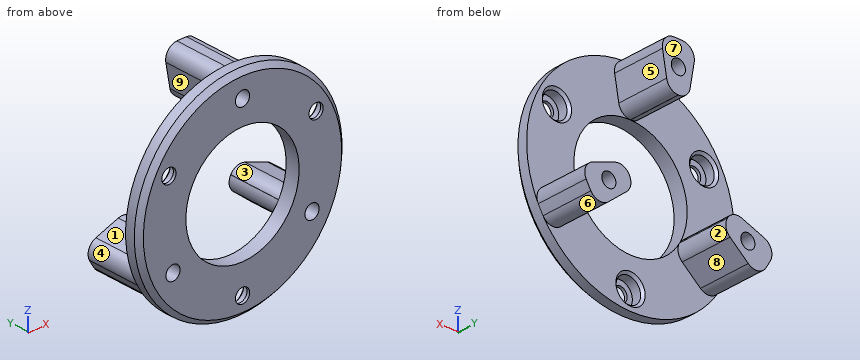
from build123d import *
from build123d.topology import SkipClean

# Parameters (mm, degrees)
SKETCH1_R           = 22
SKETCH1_R_2         = 12
BOSS_EXTRUDE1_DEPTH = 3
SKETCH3_R           = 1.5
CUT_EXTRUDE2_DEPTH  = 32.256999216
SKETCH5_R           = 2.6
CUT_EXTRUDE3_DEPTH  = 2.4
CIRPATTERN1_COUNT   = 3
SKETCH4_R           = 1.5
BOSS_EXTRUDE2_DEPTH = 11
CIRPATTERN2_COUNT   = 3
FILLET1_R           = 2.5
CHAMFER1_SIZE       = 0.5
CHAMFER2_SIZE       = 1


with BuildPart() as part:
    # Sketch1 → Boss-Extrude1 (new body)
    with BuildSketch(Plane(origin=(0, 0, 0), x_dir=(1, 0, 0), z_dir=(0, 1, 0))):
        with Locations(Location((0, 0, 0), (0, 0, 270))):
            Circle(SKETCH1_R)
        with Locations(Location((0, 0, 0), (0, 0, 270))):
            Circle(SKETCH1_R_2, mode=Mode.SUBTRACT)
    extrude(amount=BOSS_EXTRUDE1_DEPTH)

    # Sketch3 → Cut-Extrude2 (cut, through all)
    with BuildSketch(Plane(origin=(0, 3, 0), x_dir=(1, 0, 0), z_dir=(0, 1, 0))):
        with Locations(Location((14.722431864, 8.5, 0), (0, 0, 270))):
            Circle(SKETCH3_R)
        with Locations(Location((0, 18, 0), (0, 0, 270))):
            Circle(SKETCH3_R)
    cut_extrude2 = extrude(amount=-CUT_EXTRUDE2_DEPTH, mode=Mode.SUBTRACT)

    # Sketch5 → Cut-Extrude3 (cut)
    with BuildSketch(Plane(origin=(0, 3, 0), x_dir=(1, 0, 0), z_dir=(0, 1, 0))):
        with Locations(Location((0, 18, 0), (0, 0, 270))):
            Circle(SKETCH5_R)
    cut_extrude3 = extrude(amount=-CUT_EXTRUDE3_DEPTH, mode=Mode.SUBTRACT)

    # CirPattern1: Cut-Extrude2, Cut-Extrude3 ×3 about axis
    cirpattern1_axis = Axis((0, 0, 0), (0, 1, 0))
    add([cut_extrude2.rotate(cirpattern1_axis, i * 360 / CIRPATTERN1_COUNT) for i in range(1, CIRPATTERN1_COUNT)], mode=Mode.SUBTRACT)
    add([cut_extrude3.rotate(cirpattern1_axis, i * 360 / CIRPATTERN1_COUNT) for i in range(1, CIRPATTERN1_COUNT)], mode=Mode.SUBTRACT)

    # Sketch4 → Boss-Extrude2 (add)
    with SkipClean():  # the faces are left unmerged after this step: merging them gives an invalid solid
        with BuildSketch(Plane(origin=(0, 3, 0), x_dir=(1, 0, 0), z_dir=(0, 1, 0))):
            with BuildLine():
                Line((9.192533317, 7.713451316), (16.852977749, 14.141327413))
                ThreePointArc((16.852977749, 14.141327413), (19.052558883, 11), (20.673237657, 7.524443153))
                Line((20.673237657, 7.524443153), (11.276311449, 4.10424172))
                ThreePointArc((11.276311449, 4.10424172), (10.392304845, 6), (9.192533317, 7.713451316))
            make_face()
            with Locations(Location((14.722431864, 8.5, 0), (0, 0, 270))):
                Circle(SKETCH4_R, mode=Mode.SUBTRACT)
        boss_extrude2 = extrude(amount=BOSS_EXTRUDE2_DEPTH)

    # CirPattern2: Boss-Extrude2 ×3 about axis
    with SkipClean():  # the faces are left unmerged after this step: merging them gives an invalid solid
        cirpattern2_axis = Axis((0, 0, 0), (0, 1, 0))
        for i in range(1, CIRPATTERN2_COUNT):
            add(boss_extrude2.rotate(cirpattern2_axis, i * 360 / CIRPATTERN2_COUNT))

    # Fillet1
    # the kernel refuses this fillet: 2.5 mm, written as the material it takes off along each edge
    with BuildSketch(Plane(origin=(9.192533317, 3, -7.713451316), x_dir=(0.7660444431189769, 0, -0.6427876096865408), z_dir=(0, 1, 0)), Plane(origin=(-11.276311449, 3, -4.10424172), x_dir=(-0.9396926207859091, 0, -0.34202014332566705), z_dir=(0, 1, 0)), Plane(origin=(2.083778132, 3, 11.817693036), x_dir=(0.1736481776669318, 0, 0.9848077530122079), z_dir=(0, 1, 0))) as fillet1_piece_1:
        with BuildLine():
            CenterArc((2.282856857, -2.5), FILLET1_R, 90, 80.071808158)
            ThreePointArc((-0.17970467, -2.068965517), (-0.045010582, -1.03837759), (0, 0))
            Line((0, 0), (2.282856857, 0))
        make_face()
    extrude(amount=16.707142143, mode=Mode.SUBTRACT)
    with BuildSketch(Plane(origin=(11.276311449, 3, -4.10424172), x_dir=(0.9396926207859079, 0, -0.34202014332567005), z_dir=(0, 1, 0)), Plane(origin=(-9.192533317, 3, -7.713451316), x_dir=(-0.7660444431189779, 0, -0.6427876096865395), z_dir=(0, 1, 0)), Plane(origin=(-2.083778132, 3, 11.817693036), x_dir=(-0.17364817766692894, 0, 0.9848077530122082), z_dir=(0, 1, 0))) as fillet1_piece_2:
        with BuildLine():
            CenterArc((2.282856857, 2.5), FILLET1_R, 189.928191842, 80.071808158)
            ThreePointArc((-0.17970467, 2.068965517), (-0.045010582, 1.03837759), (0, 0))
            Line((0, 0), (2.282856857, 0))
        make_face()
    extrude(amount=16.707142143, mode=Mode.SUBTRACT)
    with BuildSketch(Plane(origin=(20.673237657, 3, -7.524443153), x_dir=(-0.40167516398546327, 0, -0.9157822135405619), z_dir=(0, 1, 0)), Plane(origin=(-16.852977749, 3, -14.141327413), x_dir=(-0.5922530792673408, 0, 0.8057520028509721), z_dir=(0, 1, 0)), Plane(origin=(-3.820259909, 3, 21.665770566), x_dir=(0.9939282432528036, 0, 0.11003021068958989), z_dir=(0, 1, 0))) as fillet1_piece_3:
        with BuildLine():
            CenterArc((2.66576178, 2.494836964), FILLET1_R, 176.317057086, 97.365885829)
            Line((0.170924817, 2.655425023), (0, 0))
            ThreePointArc((0, 0), (1.41317492, -0.04543472), (2.826349839, 0))
        make_face()
    extrude(amount=18.065874598, mode=Mode.SUBTRACT)
    with BuildSketch(Plane(origin=(16.852977749, 3, -14.141327413), x_dir=(0.5922530792673405, 0, 0.8057520028509723), z_dir=(0, 1, 0)), Plane(origin=(-20.673237657, 3, -7.524443153), x_dir=(0.40167516398546094, 0, -0.9157822135405629), z_dir=(0, 1, 0)), Plane(origin=(3.820259909, 3, 21.665770566), x_dir=(-0.9939282432528035, 0, 0.11003021068959112), z_dir=(0, 1, 0))) as fillet1_piece_4:
        with BuildLine():
            CenterArc((2.66576178, -2.494836964), FILLET1_R, 86.317057086, 97.365885829)
            Line((0.170924817, -2.655425023), (0, 0))
            ThreePointArc((0, 0), (1.41317492, 0.04543472), (2.826349839, 0))
        make_face()
    extrude(amount=18.065874598, mode=Mode.SUBTRACT)

    # Chamfer1
    chamfer1_edges = [part.edges().sort_by_distance(p)[0] for p in [
        (0, 3, -20.6),
        (17.840123318, 3, 10.3),
        (-17.840123318, 3, 10.3),
    ]]
    chamfer(chamfer1_edges, length=CHAMFER1_SIZE)

    # Chamfer2
    chamfer2_edges = [part.edges().sort_by_distance(p)[0] for p in [
        (0, 0, -22),
    ]]
    chamfer(chamfer2_edges, length=CHAMFER2_SIZE)


solid = part.part
Input: part model. Units: mm. Frame: model coordinates. Face numbers are marked on the shaded views. A direction names the side the tool comes from. Round coordinates to 2 decimals unless told otherwise and drop trailing zeros. Answer as CSV lines item,"result". Start each with the question number.
(1) Reachability of the marked faces 1, 2, 3, 4 and 5 from +Z, -Z, +X, -X, +Y, -Y: full face, straight path, thin tool, end or side. Return the list, or none.
(2) Line query: line 1 (X direction, y = 1, z = -8); line 2 (X direction, y = 1.7, z = 9); line 3 (Y direction, x = -9, z = -8.5). Output: solid intervals per line, ascending. Write a range as [from, to].
(3) Section A-A, the plane y = 12.5. State how many separate pieces and enclosed holes the cut face has, plus the area to 3 significant figures.
(4) First-contact query: pin 1 (2.5 mm diameter, centred on x = -15, z = 8.5, fed in from +Y); pin 2 (3 mm diameter, centred on x = 16, y = 6.5, fed in from +Z); pin 3 (5 mm diameter, centred on x = -4.5, y = 1.5, fed in from +Z). Flat tips, straight axial feed; report the tip coordinate or a pass-through.
(5) Draft query along X for the marked faces 6, 7, 8 and 9. Return one class per face: released by +X, released by -X, zero draft, split by the parting line, or undercut.
Values found:
1,face 1,"+Z, -X, +Y"
1,face 2,"+Y"
1,face 3,"+Z, +Y"
1,face 4,"-X, +Y"
1,face 5,"-Z, +X, +Y"
2,line 1,"x = [-20.49, -16.14], [-13.31, -8.94], [8.94, 13.31], [16.14, 20.49]"
2,line 2,"x = [-20.07, -18.19], [-12.99, -7.94], [7.94, 12.99], [18.19, 20.07]"
2,line 3,"y = [0, 3]"
3,separate pieces,"3"
3,enclosed holes,"3"
3,area,"141 mm²"
4,pin 1,"stops at y = 0.6"
4,pin 2,"stops at z = -5.28"
4,pin 3,"stops at z = 21.91"
5,face 6,"undercut"
5,face 7,"zero draft"
5,face 8,"undercut"
5,face 9,"released by -X"
